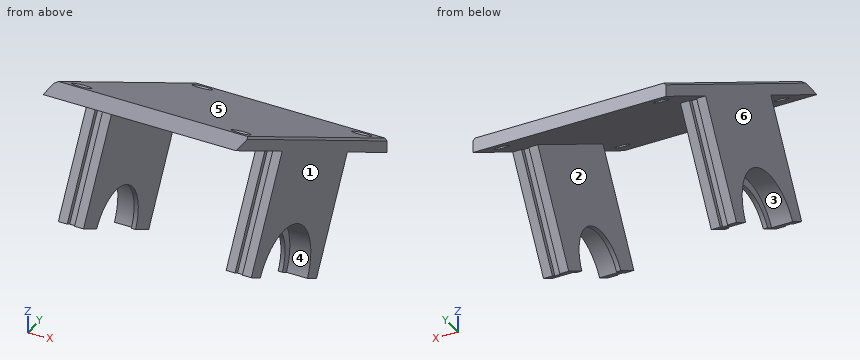
from build123d import *

# Parameters (mm, degrees)
BOSS_EXTRUDE1_DEPTH = 46
SKETCH2_R           = 1.7
CUT_EXTRUDE1_DEPTH  = 46
BOSS_EXTRUDE3_DEPTH = 27.5
SKETCH8_R           = 12.1
CUT_EXTRUDE2_DEPTH  = 63.75
BOSS_EXTRUDE4_START = -5
BOSS_EXTRUDE4_DEPTH = 1
BOSS_EXTRUDE5_START = -41
BOSS_EXTRUDE5_DEPTH = 1
CHAMFER1_SIZE       = 0.5


# Read off the part's stored shape, not the designer's step: Boss-Extrude5
with BuildPart() as part:
    # Sketch1 → Boss-Extrude1 (new body)
    with BuildSketch(Plane(origin=(0, 0, 0), x_dir=(0, 0, -1), z_dir=(1, 0, 0))):
        Polygon((0, 0), (0, 6), (35.345898385, 67.220891842), (38.81, 67.220891842), align=None)
    extrude(amount=BOSS_EXTRUDE1_DEPTH)

    # Sketch2 → Cut-Extrude1 (cut)
    with BuildSketch(Plane(origin=(0, 1.5, 2.598076211), x_dir=(1, 0, 0), z_dir=(0, 0.4999999999999947, 0.8660254037844417))):
        with Locations(Location((4, 9.5, 0), (0, 0, 270))):
            Circle(SKETCH2_R)
        with Locations(Location((42, 9.5, 0), (0, 0, 270))):
            Circle(SKETCH2_R)
        with Locations(Location((42, 71.5, 0), (0, 0, 270))):
            Circle(SKETCH2_R)
        with Locations(Location((4, 71.5, 0), (0, 0, 270))):
            Circle(SKETCH2_R)
    extrude(amount=-CUT_EXTRUDE1_DEPTH, mode=Mode.SUBTRACT)

    # Sketch7 → Boss-Extrude3 (add)
    with BuildSketch(Plane(origin=(0, 0, 0), x_dir=(-1, 0, 0), z_dir=(0, -0.49999999999999495, -0.8660254037844417))):
        Polygon((-42.125, 23.75), (-40, 23.75), (-40, 57.25), (-42.125, 57.25), (-42.125, 56), (-43.875, 56), (-43.875, 57.25), (-46, 57.25), (-46, 23.75), (-43.875, 23.75), (-43.875, 25), (-42.125, 25), align=None)
        Polygon((-6, 57.25), (-6, 23.75), (-3.875, 23.75), (-3.875, 25), (-2.125, 25), (-2.125, 23.75), (0, 23.75), (0, 57.25), (-2.125, 57.25), (-2.125, 56), (-3.875, 56), (-3.875, 57.25), align=None)
    extrude(amount=BOSS_EXTRUDE3_DEPTH)

    # Sketch8 → Cut-Extrude2 (cut)
    with BuildSketch(Plane(origin=(46, 0, 0), x_dir=(0, 0, -1), z_dir=(1, 0, 0))):
        with Locations((44.256224193, 21.214028853)):
            Circle(SKETCH8_R)
    extrude(amount=-CUT_EXTRUDE2_DEPTH, mode=Mode.SUBTRACT)

    # Sketch9 → Boss-Extrude4 (add)
    with BuildSketch(Plane(origin=(46, 0, 0), x_dir=(0, 0, -1), z_dir=(1, 0, 0)).offset(BOSS_EXTRUDE4_START)):
        with BuildLine():
            ThreePointArc((50.114698521, 31.801204045), (33.777316807, 27.264028853), (38.016698687, 10.846853661))
            Line((38.016698687, 10.846853661), (39.066908751, 12.665870851))
            ThreePointArc((39.066908751, 12.665870851), (35.595970155, 26.214028853), (49.064488458, 29.982186856))
            Line((49.064488458, 29.982186856), (50.114698521, 31.801204045))
        make_face()
    extrude(amount=-BOSS_EXTRUDE4_DEPTH)

    # Boss-Extrude5 outline → Boss-Extrude5 (add)
    with BuildSketch(Plane(origin=(46, 0, 0), x_dir=(0, 0, -1), z_dir=(1, 0, 0)).offset(BOSS_EXTRUDE5_START)):
        with BuildLine():
            ThreePointArc((39.066908751, 12.665870851), (35.595970155, 26.214028854), (49.064488458, 29.982186856))
            Line((49.064488458, 29.982186856), (50.114698521, 31.801204045))
            ThreePointArc((50.114698521, 31.801204045), (33.777316807, 27.264028853), (38.016698687, 10.846853661))
            Line((38.016698687, 10.846853661), (39.066908751, 12.665870851))
        make_face()
    extrude(amount=BOSS_EXTRUDE5_DEPTH)

    # Chamfer1
    chamfer1_edges = [part.edges().sort_by_distance(p)[0] for p in [
        (46, 36.610445921, -17.672949192),
        (4, 64.893059557, -34.001923789),
        (42, 64.893059557, -34.001923789),
        (42, 11.199484522, -3.001923789),
        (4, 11.199484522, -3.001923789),
        (0, 36.610445921, -17.672949192),
    ]]
    chamfer(chamfer1_edges, length=CHAMFER1_SIZE)


solid = part.part
Design review of the part built by this model. Coordinates are the model's own, in mm. Face numbers are marked on the shaded views. A direction names the side the tool comes from. Round coordinates to 2 decimals unless told otherwise and drop trailing zeros. Order: outer loops, then holes, each group sorted by start corner. A loop starts at its lowest first (then second) coordinate and runs counter-clockwise, first axis right, second up. Notation, with made-up numbers: M 41,-3.75 L 58,-3.75 A18 cw 58,30.25 Z; hole C -15.5,12 d7. An arc over 180 degrees is marked long. Answer as CSV lines item,"result". Start each with the question number.
1) Tool access review of the marked faces 1, 2 and 3: name each direction out of +Z, -Z, +X, -X, +Y, -Y from which nothing blocks a thin tool from reaching the whole face with its end or side.
2) Add section C-C (x = 30.5). Give the boundary of the cut face in (y, z).
3) Add section A-A (z = -31). Give the number of separate pieces and of enclosed holes in the cut face, then the cut area to 3 significant figures.
4) Add section D-D (z = -22). Give the boundary of the cut face in (x, y) (3 decimals), then the cut area to 3 significant figures.
5) Add section B-B (y = 47). Give the boundary of the cut face in (x, z) (3 decimals).
6) For pin 1 Ø12 at (x, y) = (16.5, 12.5) entering from +Z; pin 2 Ø10 at (x, z) = (15.5, -44) entering from +Y; pin 3 Ø1.5 at (x, y) = (33.5, 36) entering from +Z; pin 4 Ø10 at (x, y) = (31, 15) entering from +Z, all flat-tipped, find the tip position at first contact; note any pin that passes through.
7) Wall thickness on line 1 along X through (y, z) = (12, -35); line 2 along Y through (x, z) = (2, -8); line 3 along Y through (x, z) = (10, -7): over which ranges is each line inside the solid? List them lowest first. Write a range as [from, to].
8) The part is to be moulded in two halves that separate along Y. For the marked faces 4, 5 and 6, say which applies: +Y half, -Y half, draft (parallel to the pull), parting line (faces both ways), or undercut.
Resolved:
1,face 1,"+Z, -Z, +X, +Y, -Y"
1,face 2,"-Z, -Y"
1,face 3,"-X"
2,outline,"M 0,0 L 67.22,-38.81 L 67.22,-35.35 L 6,0 Z"
3,separate pieces,"3"
3,enclosed holes,"0"
3,area,"730 mm^2"
4,outline,"M 0,14.722 L 2.125,14.722 L 2.125,16.166 L 3.875,16.166 L 3.875,14.722 L 6,14.722 L 6,38.105 L 40,38.105 L 40,14.722 L 42.125,14.722 L 42.125,16.166 L 43.875,16.166 L 43.875,14.722 L 46,14.722 L 46,43.105 L 45.5,44.105 L 0.5,44.105 L 0,43.105 Z"
4,area,"551 mm^2"
5,outline,"M 0,-33.094 L 2.125,-33.094 L 2.125,-30.594 L 3.875,-30.594 L 3.875,-33.094 L 6,-33.094 L 6,-27.135 L 40,-27.135 L 40,-33.094 L 42.125,-33.094 L 42.125,-30.594 L 43.875,-30.594 L 43.875,-33.094 L 46,-33.094 L 46,-24.249 L 45.5,-23.671 L 0.5,-23.671 L 0,-24.249 Z"
6,pin 1,"z = -0.29"
6,pin 2,"through"
6,pin 3,"z = -16.89"
6,pin 4,"z = -2.31"
7,line 1,"[0, 6], [40, 46]"
7,line 2,"[13.86, 19.86]"
7,line 3,"[12.12, 18.12]"
8,face 4,"undercut"
8,face 5,"+Y half"
8,face 6,"draft"
